The drawing under review shows one solid part. Ordinate dimensions are in mm from its lowest x, y, z. Give positions to 0.01 mm unless a question says otherwise; leave off trailing zeros. Write each loop counter-clockwise with the first axis right and the second up, starting at its lowest first coordinate (ties: lowest second). Pieces come first, ordered by that corner, then holes. Notation, with made-up numbers: M 71.5,-24 L 124.5,-24 A21 ccw 124.5,4 Z; hole C 60,70.5 d11. An arc over 180 degrees is marked long. Write item = value, one per line. Start each with the question number.
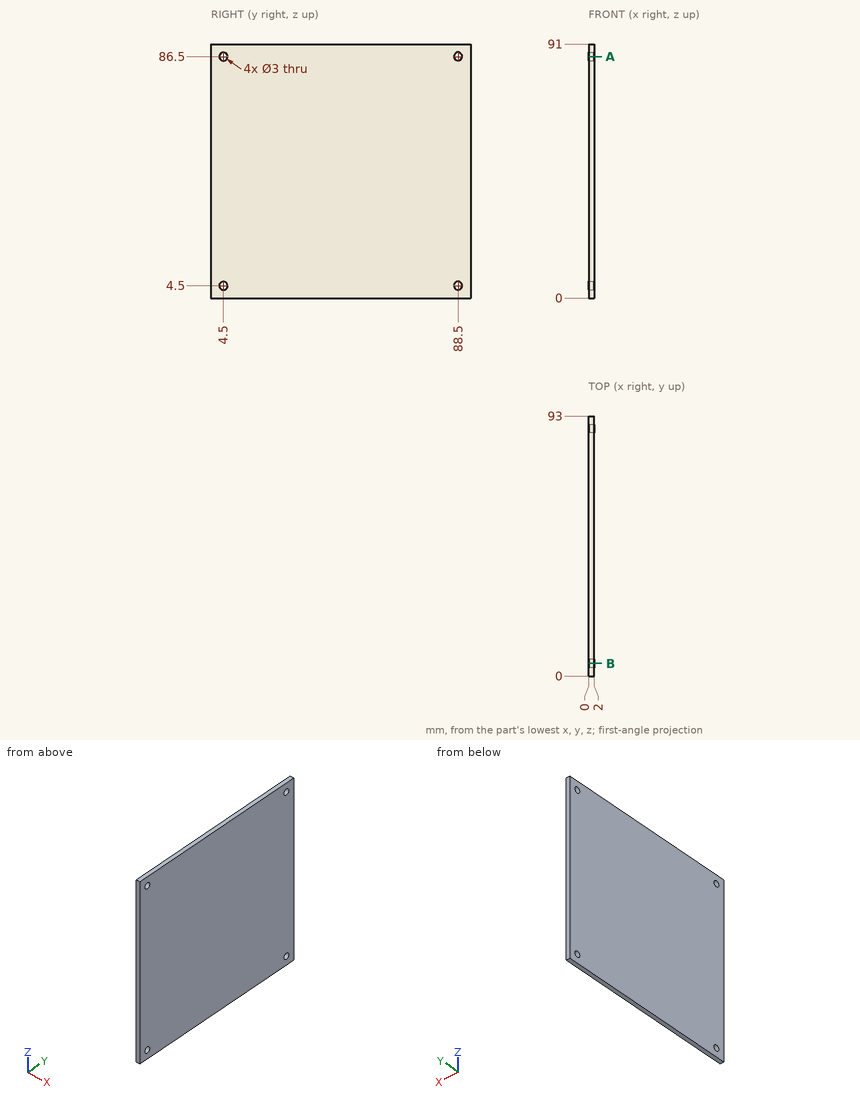
Item 1: To check wall thickness, follow probe 1 along Y at (x, z) = (1.25, 86.5); probe 2 along Z at (x, y) = (1.4, 88.5). State the ranges of each line that lie inside material, in increasing order. Write a range as [from, to].
Item 2: We need section B-B, the plane y = 4.5. Write out the cut boundary in (x, z).
Item 3: We need section A-A, the plane z = 86.5. Write out the cut boundary in (x, y), and give its area (3 significant figures).
Worked out:
q1.probe_1 = [0, 3], [6, 87], [90, 93]
q1.probe_2 = [0, 3], [6, 85], [88, 91]
q2.outline = M 0,0 L 2,0 L 2,3 L 0,3 Z; M 0,6 L 2,6 L 2,85 L 0,85 Z; M 0,88 L 2,88 L 2,91 L 0,91 Z
q3.outline = M 0,0 L 2,0 L 2,3 L 0,3 Z; M 0,6 L 2,6 L 2,87 L 0,87 Z; M 0,90 L 2,90 L 2,93 L 0,93 Z
q3.area = 174 mm²
